Input: part model. Units: mm. Frame: model coordinates. Coordinates: 2 decimals unless noted, no trailing zeros. Use CSV: the item, a comma, the result in double quotes.
```python
from build123d import *

# Parameters (mm, degrees)
SKETCH041_W      = 125
SKETCH041_H      = 96
EXTRUDE024_DEPTH = 3
SKETCH042_R      = 1.6
HOLE016_DEPTH    = 3
HOLE016_TIPS_R   = 1.6
FILLET002_R      = 2


with BuildPart() as part:
    # Sketch041 → Extrude024 (new body)
    with BuildSketch(Plane.XY):
        with Locations((15.050004, 71.699999)):
            Rectangle(SKETCH041_W, SKETCH041_H)
    extrude(amount=-EXTRUDE024_DEPTH)

    # Sketch042 (on Face6 of BaseFeature004) → Hole016 (cut)
    with BuildSketch(Plane(origin=(0, 0, -3), x_dir=(1, 0, 0), z_dir=(0, 0, -1))):
        with Locations((-31.331001, -31.335001)):
            Circle(SKETCH042_R)
        with Locations((-31.332001, -112.083005)):
            Circle(SKETCH042_R)
        with Locations((61.449498, -112.077997)):
            Circle(SKETCH042_R)
        with Locations((61.460003, -31.285001)):
            Circle(SKETCH042_R)
    extrude(amount=-HOLE016_DEPTH, mode=Mode.SUBTRACT)

    # Hole016 tips → Hole016 tip 1 section 0
    with BuildSketch(Plane(origin=(0, 0, 0), x_dir=(1, 0, 0), z_dir=(0, 0, -1)), mode=Mode.PRIVATE) as hole016_tip_1_s0:
        with Locations((-31.331001, -31.335001)):
            Circle(HOLE016_TIPS_R)
    loft([hole016_tip_1_s0.sketch, Vertex(-31.331001, 31.335001, 0.961377)], mode=Mode.SUBTRACT)

    # Hole016 tips → Hole016 tip 2 section 0
    with BuildSketch(Plane(origin=(0, 0, 0), x_dir=(1, 0, 0), z_dir=(0, 0, -1)), mode=Mode.PRIVATE) as hole016_tip_2_s0:
        with Locations((-31.332001, -112.083005)):
            Circle(HOLE016_TIPS_R)
    loft([hole016_tip_2_s0.sketch, Vertex(-31.332001, 112.083005, 0.961377)], mode=Mode.SUBTRACT)

    # Hole016 tips → Hole016 tip 3 section 0
    with BuildSketch(Plane(origin=(0, 0, 0), x_dir=(1, 0, 0), z_dir=(0, 0, -1)), mode=Mode.PRIVATE) as hole016_tip_3_s0:
        with Locations((61.449498, -112.077997)):
            Circle(HOLE016_TIPS_R)
    loft([hole016_tip_3_s0.sketch, Vertex(61.449498, 112.077997, 0.961377)], mode=Mode.SUBTRACT)

    # Hole016 tips → Hole016 tip 4 section 0
    with BuildSketch(Plane(origin=(0, 0, 0), x_dir=(1, 0, 0), z_dir=(0, 0, -1)), mode=Mode.PRIVATE) as hole016_tip_4_s0:
        with Locations((61.460003, -31.285001)):
            Circle(HOLE016_TIPS_R)
    loft([hole016_tip_4_s0.sketch, Vertex(61.460003, 31.285001, 0.961377)], mode=Mode.SUBTRACT)

    # Fillet002
    fillet002_edges = [part.edges().sort_by_distance(p)[0] for p in [
        (-47.449996, 23.699999, -1.5),
        (-47.449996, 71.699999, -3),
        (15.050004, 23.699999, -3),
        (77.550004, 23.699999, -1.5),
        (77.550004, 71.699999, -3),
        (77.550004, 119.699999, -1.5),
        (15.050004, 119.699999, -3),
        (-47.449996, 119.699999, -1.5),
    ]]
    fillet(fillet002_edges, radius=FILLET002_R)


with BuildPart() as part_1:
    # Body003 placement: moved
    add(part.part.moved(Location((0, 0, -41.83))))


solid = part_1.part
```
1. Section A-A (z = -44.3). State how many separate pieces and enclosed holes the cut face has, then the cut area to 3 significant figures.
Resolved:
separate pieces,"1"
enclosed holes,"4"
area,"11,700 mm^2"
2. Contact query for a flat-ended pin moving along its axis: pin 1 Ø4 at (x, y) = (-31.33, 112.08) entering from -Z. Output: stop coordinate, or through.
Resolved:
pin 1,"stops at z = -44.83"
3. Mould query, pull axis X, two halves, no side actions, for faces 1 (the cylindrical face through (-30.472, 110.734, -43.351)), 2 (the flat face through (14, 72, -44.83)). Classes: pulls with the +X half, pulls with the -X half, needs draft (parallel to the pull), parting line crosses it, or undercut.
Resolved:
face 1,"undercut"
face 2,"needs draft"
4. Material intervals for line 1 (X direction, y = 32.5, z = -42.85); line 2 (X direction, y = 32, z = -44); line 3 (Y direction, x = 57, z = -43.15), sorted ascending. Write a range as [from, to].
Resolved:
line 1,"x = [-47.45, -32.43], [-30.23, 60.42], [62.5, 77.55]"
line 2,"x = [-47.07, -32.79], [-29.88, 60.03], [62.89, 77.17]"
line 3,"y = [23.73, 119.67]"
